The model under review builds one solid part; all positions refer to its coordinate system, in mm. Face numbers are marked on the shaded views. A direction names the side the tool comes from. Give positions to 0.01 mm unless a question says otherwise; leave off trailing zeros. Order: outer loops, then holes, each group sorted by start corner. A loop starts at its lowest first (then second) coordinate and runs counter-clockwise, first axis right, second up. Notation, with made-up numbers: (13.25, 3.25) - (52.25, 3.25) arc R16 ccw to (52.25, 34.25) - close; hole circle Ø7 at (-5.75, -0.5). An arc over 180 degrees is marked (long way). Put each result on its own line as item: value.
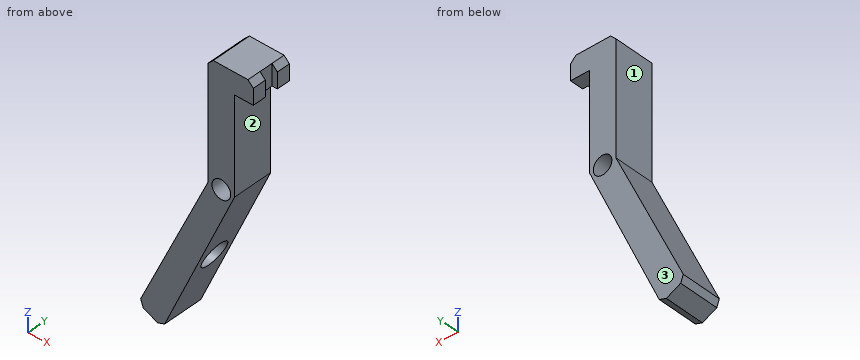
```python
from build123d import *

# Parameters (mm, degrees)
F0_R        = 1.75
F1_DEPTH    = 7.5
F2_T1_DEPTH = 12.6433659759
F2_T3_DEPTH = 12.7137209508
F3_R        = 2.5
F4_DEPTH    = 5
F5_W        = 2.5
F5_H        = 3
F6_DEPTH    = 1
F7_W        = 1
F7_H        = 2.5
F8_DEPTH    = 25


# Not quite as in the source:
# - a fillet or chamfer that OpenCascade refuses, or shapes differently, is made with other operations: its cross-section is extruded or revolved along the edge and cut away or added


with BuildPart() as f1:
    # F0 (on Front) → F1 (new body)
    with BuildSketch(Plane.XZ):
        Polygon((-29.1562567131, -15.4619954874), (-25.6562567131, -15.4619954874), (-25.6562567131, -11.4619954874), (-34.1562567131, -11.4619954874), (-34.1562567131, -33.4619954874), (-47.2335256009, -61.5062891187), (-42.7019866657, -63.6193804274), (-29.1562567131, -33.4619954874), align=None)
        with Locations((-31.6562567131, -33.4619954874)):
            Circle(F0_R, mode=Mode.SUBTRACT)
    extrude(amount=F1_DEPTH)

    # F2: chamfer of 1 on 4 edges, made by hand

    # F2_s2 → F2_t1 (cut)
    with BuildSketch(Plane.XZ.offset(-2.571682988)):
        Polygon((-33.1562567131, -11.4619954874), (-34.1562567131, -12.4619954874), (-34.1562567131, -11.4619954874), align=None)
        Polygon((-25.6562567131, -12.4619954874), (-26.6562567131, -11.4619954874), (-25.6562567131, -11.4619954874), align=None)
        Polygon((-46.8109073392, -60.5999813317), (-46.3272178139, -61.9289073804), (-47.2335256009, -61.5062891187), align=None)
    extrude(amount=F2_T1_DEPTH, mode=Mode.SUBTRACT)

    # F2_s4 → F2_t3 (cut)
    with BuildSketch(Plane.XZ.offset(-2.6068604754)):
        Polygon((-42.2864056117, -62.6941561786), (-43.6212292029, -63.1907305926), (-42.7019866657, -63.6193804274), align=None)
    extrude(amount=F2_T3_DEPTH, mode=Mode.SUBTRACT)

    # F3 (on face) → F4 (cut)
    with BuildSketch(Plane(origin=(-34.1562567131, 0, 0), x_dir=(0, -1, 0), z_dir=(-1, 0, 0))):
        with Locations((3.75, -49.4619954874)):
            Circle(F3_R)
    extrude(amount=F4_DEPTH, mode=Mode.SUBTRACT)

    # F5 (on face) → F6 (cut)
    with BuildSketch(Plane.YZ.offset(-25.6562567131)):
        with Locations((-3.75, -13.9619954874)):
            Rectangle(F5_W, F5_H)
    extrude(amount=-F6_DEPTH, mode=Mode.SUBTRACT)

    # F7 (on face) → F8 (cut)
    with BuildSketch(Plane(origin=(0, 0, -12.4619954874), x_dir=(1, 0, 0), z_dir=(0, 0, -1))):
        with Locations((-26.1562567131, 3.75)):
            Rectangle(F7_W, F7_H)
    extrude(amount=-F8_DEPTH, mode=Mode.SUBTRACT)


solid = f1.part
```
(1) For the marked faces 1, 2 and 3, list the 3-axis set-ups (+Z, -Z, +X, -X, +Y, -Y) from which the entire face can be reached by the end or side of a thin tool; tool diameter is ignored.
The answers:
face 1: +Z, -X, +Y, -Y
face 2: -Z, +X, +Y, -Y
face 3: +Z, -Z, +X, -X, +Y
(2) Take a section at A-A, the plane z = -14.5. Write out the cut boundary in (x, y), then the cut area to 4 significant figures.
The answers:
outline: (-34.16, -7.5) - (-25.66, -7.5) - (-25.66, -5) - (-26.66, -5) - (-26.66, -2.5) - (-25.66, -2.5) - (-25.66, 0) - (-34.16, 0) - close
area: 61.25 mm^2
(3) Clearance check with flat-ended pins moving along their axes: pin 1 Ø3 at (y, z) = (-4.5, -36) entering from -X; pin 2 Ø1.5 at (x, z) = (-37.5, -37) entering from -Y; pin 3 Ø4.5 at (x, z) = (-31.66, -33.46) entering from +Y; pin 4 Ø3 at (y, z) = (-3, -17.5) entering from -X. State where each tip first meets the part, or that it passes through.
The answers:
pin 1: x = -36.04
pin 2: through
pin 3: y = 0
pin 4: x = -34.16
(4) Wall thickness on L1, parallel to Z at x = -27.5, y = -3; L2, parallel to X at y = -3.5, z = -25.5; L3, parallel to Z at x = -38.5, y = -4.5: over which ranges is each line inside the solid? List them lowest first.
The answers:
L1: -15.46 to -11.46
L2: -34.16 to -29.16
L3: -54.26 to -51.85, -47.08 to -42.78
(5) Take a section at D-D, the plane z = -53.5. Write out the cut boundary in (x, y).
The answers:
outline: (-43.5, -7.5) - (-38.16, -7.5) - (-38.16, 0) - (-43.5, 0) - close
(6) Take a section at B-B, the plane y = -3.75. Write out the cut boundary in (x, z).
The answers:
outline: (-46.81, -60.6) - (-46.33, -61.93) - (-43.62, -63.19) - (-42.29, -62.69) - (-37.47, -51.96) - (-39.16, -51.96) - (-39.16, -46.96) - (-35.22, -46.96) - (-29.16, -33.46) - (-29.16, -15.46) - (-26.66, -15.46) - (-26.66, -11.46) - (-33.16, -11.46) - (-34.16, -12.46) - (-34.16, -33.46) - close; hole circle Ø3.5 at (-31.66, -33.46)
(7) Take a section at C-C, the plane x = -28.5. Write out the cut boundary in (y, z).
The answers:
outline: (-7.5, -15.46) - (0, -15.46) - (0, -11.46) - (-7.5, -11.46) - close
